```python
from build123d import *

# Parameters (mm, degrees)
SKETCH1_W            = 50
SKETCH1_H            = 175
BOSS_EXTRUDE1_DEPTH  = 9
SKETCH2_R            = 6
CUT_EXTRUDE1_DEPTH   = 92.445338864
BOSS_EXTRUDE2_DEPTH  = 9
BOSS_EXTRUDE3_START  = 3
BOSS_EXTRUDE3_DEPTH  = 12
FILLET1_R            = 9
FILLET1_OF_MIRROR4_R = 9


with BuildPart() as part:
    # Sketch1 → Boss-Extrude1 (new body)
    with BuildSketch(Plane(origin=(0, 0, 0), x_dir=(1, 0, 0), z_dir=(0, 1, 0))):
        Rectangle(SKETCH1_W, SKETCH1_H)
    extrude(amount=BOSS_EXTRUDE1_DEPTH)

    # Sketch2 → Cut-Extrude1 (cut, through all)
    with BuildSketch(Plane(origin=(0, 9, 0), x_dir=(1, 0, 0), z_dir=(0, 1, 0))):
        with Locations(Location((0, -71.5, 0), (0, 0, 270))):
            Circle(SKETCH2_R)
    cut_extrude1 = extrude(amount=-CUT_EXTRUDE1_DEPTH, mode=Mode.SUBTRACT)

    # Mirror1: Cut-Extrude1 across plane
    add(cut_extrude1.mirror(Plane.XY), mode=Mode.SUBTRACT)

    # Sketch3 → Boss-Extrude2 (add)
    with BuildSketch(Plane(origin=(25, 0, 0), x_dir=(0, 0, -1), z_dir=(1, 0, 0))):
        with BuildLine():
            Line((-19.286429863, 52.90703062), (-55.5, 9))
            Line((-55.5, 9), (0, 9))
            Line((0, 9), (0, 12))
            ThreePointArc((0, 12), (-22.612781402, 26.338756299), (-19.286429863, 52.90703062))
        make_face()
        with BuildLine():
            Line((0, 12), (0, 9))
            Line((0, 9), (55.5, 9))
            Line((55.5, 9), (19.286429863, 52.90703062))
            ThreePointArc((19.286429863, 52.90703062), (23.528288788, 45.451013355), (25, 37))
            ThreePointArc((25, 37), (17.67766953, 19.32233047), (0, 12))
        make_face()
    boss_extrude2 = extrude(amount=-BOSS_EXTRUDE2_DEPTH)

    # Sketch3_3 → Boss-Extrude3 (add)
    with BuildSketch(Plane(origin=(25, 0, 0), x_dir=(0, 0, -1), z_dir=(1, 0, 0)).offset(BOSS_EXTRUDE3_START)):
        with BuildLine():
            ThreePointArc((0, 62), (-10.661243701, 59.612781402), (-19.286429863, 52.90703062))
            ThreePointArc((-19.286429863, 52.90703062), (-22.612781402, 26.338756299), (0, 12))
            Line((0, 12), (0, 24.5))
            ThreePointArc((0, 24.5), (-12.5, 37), (0, 49.5))
            Line((0, 49.5), (0, 62))
        make_face()
        with BuildLine():
            ThreePointArc((19.286429863, 52.90703062), (10.661243701, 59.612781402), (0, 62))
            Line((0, 62), (0, 49.5))
            ThreePointArc((0, 49.5), (8.838834765, 45.838834765), (12.5, 37))
            ThreePointArc((12.5, 37), (8.838834765, 28.161165235), (0, 24.5))
            Line((0, 24.5), (0, 12))
            ThreePointArc((0, 12), (17.67766953, 19.32233047), (25, 37))
            ThreePointArc((25, 37), (23.528288788, 45.451013355), (19.286429863, 52.90703062))
        make_face()
    boss_extrude3 = extrude(amount=-BOSS_EXTRUDE3_DEPTH)

    # Fillet1
    fillet1_edges = [part.edges().sort_by_distance(p)[0] for p in [
        (20.5, 9, -55.5),
        (20.5, 9, 55.5),
    ]]
    fillet(fillet1_edges, radius=FILLET1_R)

    # Mirror4: Boss-Extrude2, Boss-Extrude3 across plane
    add(boss_extrude2.mirror(Plane(origin=(0, 0, 0), x_dir=(0, 0, 1), z_dir=(1, 0, 0))))
    add(boss_extrude3.mirror(Plane(origin=(0, 0, 0), x_dir=(0, 0, 1), z_dir=(1, 0, 0))))

    # Fillet1 of Mirror4
    fillet1_of_mirror4_edges = [part.edges().sort_by_distance(p)[0] for p in [
        (-20.5, 9, -55.5),
        (-20.5, 9, 55.5),
    ]]
    fillet(fillet1_of_mirror4_edges, radius=FILLET1_OF_MIRROR4_R)


solid = part.part
```
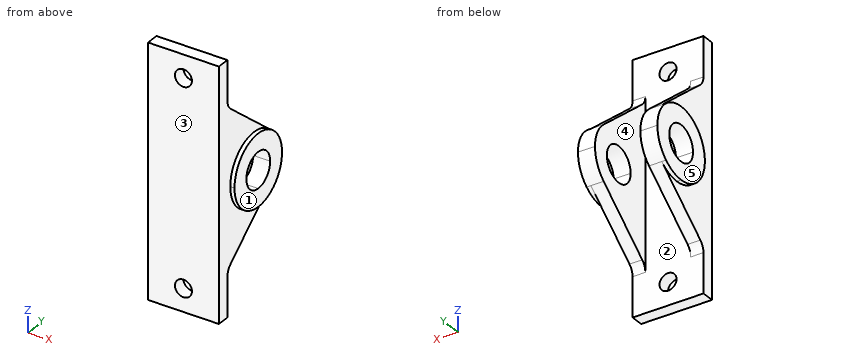
Can you work these out from the model? Positions are in its coordinate system, mm. Face numbers are marked on the shaded views. A direction names the side the tool comes from. Round coordinates to 2 decimals unless told otherwise and drop trailing zeros. Loops run counter-clockwise (first coordinate to the right, second up) from the corner with the lowest first, then second, coordinate; pieces in that order, holes last. Notation, with made-up numbers: M 28,53 L 33,53 A21 cw 33,64 Z; hole C -15.75,58.25 d11. An arc over 180 degrees is marked long. Answer as a JSON object with one key per item and string values. Group by question number.
Q1. Imagine slicing it at A-A, the plane x = 0. Please give me the cut outline in (y, z), then the cut area to 3 significant figures.
Q2. We'd pull the mould along X, two halves only. Please class the marked faces 1, 2 and 3: +X half, -X half, draft (parallel to the pull), parting line (faces both ways), or undercut.
Q3. On a 3-axis mill with a long thin cutter (end or side, diameter ignored), from which of +Z, -Z, +X, -X, +Y, -Y can I reach the whole of each face in a straight line? I mean the marked faces 4 and 5. Say none if no direction works.
Q4. Imagine slicing it at D-D, the plane y = 22. Please give me the cut outline in (x, z).
Q5. Imagine slicing it at B-B, the plane z = -71.5. Please give me the cut outline in (x, y), then the cut area to 3 significant figures.
Q6. Please list where these lines run through material, in increasing order: L1, parallel to X at y = 5.25, z = -71.5; L2, parallel to X at y = 31.5, z = -14.5; L3, parallel to Y at x = -2, z = -45.
Q7. Will these pins go through, and if not, where does the flat tip stop? pin 1 (1.5 mm diameter, centred on x = -15.5, y = 20.5, fed in from +Z); pin 2 (5 mm diameter, centred on x = -21.5, y = 13, fed in from +Z); pin 3 (12 mm diameter, centred on x = -19.5, y = 19.5, fed in from +Z); pin 4 (11 mm diameter, centred on x = 0, z = -71.5, fed in from -Y).
Q8. Imagine slicing it at C-C, the plane y = 42. Please give me the cut outline in (x, z), then the cut area to 3 significant figures.
Findings:
{
 "1": {"outline": "M 0,-87.5 L 9,-87.5 L 9,-77.5 L 0,-77.5 Z; M 0,-65.5 L 9,-65.5 L 9,65.5 L 0,65.5 Z; M 0,77.5 L 9,77.5 L 9,87.5 L 0,87.5 Z", "area": "1,360 mm2"},
 "2": {"face 1": "+X half", "face 2": "undercut", "face 3": "draft"},
 "3": {"face 4": "+Z, -Z, +Y", "face 5": "+Z, -Z, -X, +Y, -Y"},
 "4": {"outline": "M -28,-20 L -25,-20 L -25,-44.78 L -16,-44.78 L -16,44.78 L -25,44.78 L -25,20 L -28,20 Z; M 16,-44.78 L 25,-44.78 L 25,-20 L 28,-20 L 28,20 L 25,20 L 25,44.78 L 16,44.78 Z"},
 "5": {"outline": "M -25,0 L -6,0 L -6,9 L -25,9 Z; M 6,0 L 25,0 L 25,9 L 6,9 Z", "area": "342 mm2"},
 "6": {"L1": "x = -25 to -6, 6 to 25", "L2": "x = -28 to -16, 16 to 28", "L3": "y = 0 to 9"},
 "7": {"pin 1": "stops at z = 46.48", "pin 2": "stops at z = 54.77", "pin 3": "stops at z = 51.79", "pin 4": "passes through"},
 "8": {"outline": "M -28,-24.49 L -25,-24.49 L -25,-28.28 L -16,-28.28 L -16,-11.46 L -28,-11.46 Z; M -28,11.46 L -16,11.46 L -16,28.28 L -25,28.28 L -25,24.49 L -28,24.49 Z; M 16,-28.28 L 25,-28.28 L 25,-24.49 L 28,-24.49 L 28,-11.46 L 16,-11.46 Z; M 16,11.46 L 28,11.46 L 28,24.49 L 25,24.49 L 25,28.28 L 16,28.28 Z", "area": "762 mm2"}
}
